Verification items for the finished model (mm, model axes). A direction names the side the tool comes from. Round coordinates to 2 decimals unless told otherwise and drop trailing zeros. Order: outer loops, then holes, each group sorted by start corner. A loop starts at its lowest first (then second) coordinate and runs counter-clockwise, first axis right, second up. Notation, with made-up numbers: M 66.5,-39.75 L 106.5,-39.75 A21 cw 106.5,-28.75 Z; hole C 0.25,36 d9. An arc over 180 degrees is marked long. Use one line per item in the form item = value. Start each with the question number.
Item 1: Cross-section at C-C on x = -9. Enter the section's corners in (y, z).
Item 2: Go/stop test with a flat-tipped pin: pin 1 Ø9.5 at (y, z) = (-32, 27.5) entering from +X. Record where the tip stops, or that it passes through.
Item 3: Thickness scan on probe 1 along Y at (x, z) = (-12, 24.5); probe 2 along X at (y, z) = (-20, 20). Record the ranges inside material, lowest first. Write a range as [from, to].
Item 4: Tool access check on faces 1 (the flat face through (-26, -38.1, 27)), 2 (the flat face through (-16.073, -29, 27)). Record the directions out of +Z, -Z, +X, -X, +Y, -Y that give a thin tool (end or side, any length) a straight path to the whole face; none if there is none.
Item 5: Cross-section at B-B on y = -24.5. Enter the section's corners in (x, z), then the cut area to 3 significant figures.
Item 6: Cross-section at A-A on z = 30.25. Enter the section's corners in (x, y).
from build123d import *

# Parameters (mm, degrees)
F0_W     = 19.05
F0_H     = 19.05
F1_DEPTH = 38.1
F2_DEPTH = 19.05
F3_W     = 19.05
F3_H     = 19.05
F4_DEPTH = 25.4


with BuildPart() as f1:
    # F0 (on Front) → F1 (new body)
    with BuildSketch(Plane.XZ):
        with Locations((-25.597605, 27.221616)):
            Rectangle(F0_W, F0_H)
        with Locations((-6.547605, 27.221616)):
            Rectangle(F0_W, F0_H)
    extrude(amount=F1_DEPTH)

    # F0 (on Front) → F2 (join)
    with BuildSketch(Plane.XZ):
        with Locations((-6.547605, 27.221616)):
            Rectangle(F0_W, F0_H)
    extrude(amount=F2_DEPTH)

    # F3 (on face) → F4 (cut)
    with BuildSketch(Plane.XY.offset(36.746616)):
        with Locations((-6.547605, -28.575)):
            Rectangle(F3_W, F3_H)
    extrude(amount=-F4_DEPTH, mode=Mode.SUBTRACT)


solid = f1.part
Output values:
q1.outline = M -19.05,17.7 L 0,17.7 L 0,36.75 L -19.05,36.75 Z
q2.pin_1 = -16.07
q3.probe_1 = [-19.05, 0]
q3.probe_2 = [-35.12, -16.07]
q4.face_1 = +Z, -Z, +X, -X, -Y
q4.face_2 = +Z, -Z, +X, -Y
q5.outline = M -35.12,17.7 L -16.07,17.7 L -16.07,36.75 L -35.12,36.75 Z
q5.area = 363 mm2
q6.outline = M -35.12,-38.1 L -16.07,-38.1 L -16.07,-19.05 L 2.98,-19.05 L 2.98,0 L -35.12,0 Z
